The model under review builds one solid part; all positions refer to its coordinate system, in mm. Face numbers are marked on the shaded views. A direction names the side the tool comes from. Coordinates: 2 decimals unless noted, no trailing zeros. Loops run counter-clockwise (first coordinate to the right, second up) from the corner with the lowest first, then second, coordinate; pieces in that order, holes last. Notation, with made-up numbers: (-11.5, 74) - (2.5, 74) arc R19 ccw to (2.5, 107) - close; hole circle Ø3 at (26, 40). An arc over 180 degrees is marked (long way). Use a Markdown table: item, result. Add a question column.
1) Clearance check with flat-ended pins moving along their axes: pin 1 (3 mm diameter, centred on x = -34, z = -34, fed in from +Y); pin 2 (1 mm diameter, centred on y = 7.5, z = 30, fed in from -X). State where each tip first meets the part, or that it passes through.
2) For the marked faces 1 and 2, list the 3-axis set-ups (+Z, -Z, +X, -X, +Y, -Y) from which the entire face can be reached by the end or side of a thin tool; tool diameter is ignored.
3) Add section A-A, the plane z = 34. Give the boundary of the cut face in (x, y), and give its area (3 significant figures).
4) Add section B-B, the plane x = 34. Give the boundary of the cut face in (y, z).
5) To check wall thickness, follow L1, parallel to X at y = 0.4, z = 34; L2, parallel to Z at x = 35, y = 6.75; L3, parallel to Y at x = 31.5, z = -31.5. State the ranges of each line that lie inside material, in increasing order. Write a range as [from, to].
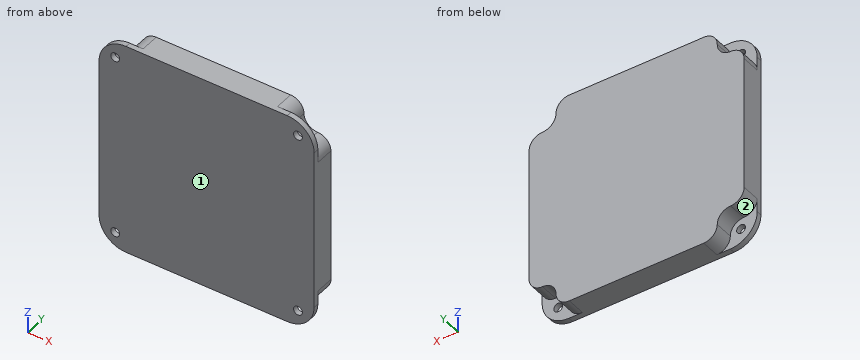
```python
from build123d import *

# Parameters (mm, degrees)
SKETCH_1_R      = 1.65
EXTRUDE_1_DEPTH = 2
EXTRUDE_2_DEPTH = 7
FILLET_1_R      = 5


with BuildPart() as part:
    # 草图1 → 凸台-拉伸1 (new body)
    with BuildSketch(Plane(origin=(0, 0, 0), x_dir=(1, 0, 0), z_dir=(0, 1, 0))):
        with BuildLine():
            Line((-30, -40), (30, -40))
            ThreePointArc((30, -40), (37.071067812, -37.071067812), (40, -30))
            Line((40, -30), (40, 30))
            ThreePointArc((40, 30), (37.071067812, 37.071067812), (30, 40))
            Line((30, 40), (-30, 40))
            ThreePointArc((-30, 40), (-37.071067812, 37.071067812), (-40, 30))
            Line((-40, 30), (-40, -30))
            ThreePointArc((-40, -30), (-37.071067812, -37.071067812), (-30, -40))
        make_face()
        with Locations(Location((-34, 34, 0), (0, 0, 270))):
            Circle(SKETCH_1_R, mode=Mode.SUBTRACT)
        with Locations(Location((-34, -34, 0), (0, 0, 90))):
            Circle(SKETCH_1_R, mode=Mode.SUBTRACT)
        with Locations(Location((34, 34, 0), (0, 0, 90))):
            Circle(SKETCH_1_R, mode=Mode.SUBTRACT)
        with Locations(Location((34, -34, 0), (0, 0, 270))):
            Circle(SKETCH_1_R, mode=Mode.SUBTRACT)
    extrude(amount=EXTRUDE_1_DEPTH)

    # 草图2 → 凸台-拉伸2 (add)
    with BuildSketch(Plane(origin=(0, 2, 0), x_dir=(1, 0, 0), z_dir=(0, 1, 0))):
        Polygon((-30, 40), (-30, 30), (-40, 30), (-40, -30), (-30, -30), (-30, -40), (30, -40), (30, -30), (40, -30), (40, 30), (30, 30), (30, 40), align=None)
    extrude(amount=EXTRUDE_2_DEPTH)

    # 圆角1
    fillet_1_edges = [part.edges().sort_by_distance(p)[0] for p in [
        (-40, 5.5, -30),
        (-30, 5.5, -30),
        (-30, 5.5, -40),
        (30, 5.5, -40),
        (30, 5.5, -30),
        (40, 5.5, -30),
        (40, 5.5, 30),
        (30, 5.5, 30),
        (30, 5.5, 40),
        (-40, 5.5, 30),
        (-30, 5.5, 30),
        (-30, 5.5, 40),
    ]]
    fillet(fillet_1_edges, radius=FILLET_1_R - 0.0001)  # a hair under: the kernel refuses the full size


solid = part.part
```
From the geometry:
| question | item | result |
|---|---|---|
| 1 | pin 1 | passes through |
| 1 | pin 2 | stops at x = -37.18 |
| 2 | face 1 | +Z, -Z, +X, -X, -Y |
| 2 | face 2 | -Z, -X, +Y |
| 3 | outline | (-39.17, 0) - (-35.65, 0) - (-35.65, 2) - (-39.17, 2) - close; (-32.35, 0) - (32.35, 0) - (32.35, 2) - (30.1, 2) - (30.1, 9) - (-30.1, 9) - (-30.1, 2) - (-32.35, 2) - close; (35.65, 0) - (39.17, 0) - (39.17, 2) - (35.65, 2) - close |
| 3 | area | 565 mm^2 |
| 4 | outline | (0, -39.17) - (2, -39.17) - (2, -35.65) - (0, -35.65) - close; (0, -32.35) - (2, -32.35) - (2, -30.1) - (9, -30.1) - (9, 30.1) - (2, 30.1) - (2, 32.35) - (0, 32.35) - close; (0, 35.65) - (2, 35.65) - (2, 39.17) - (0, 39.17) - close |
| 5 | L1 | x = [-39.17, -35.65], [-32.35, 32.35], [35.65, 39.17] |
| 5 | L2 | z = [-30, 30] |
| 5 | L3 | y = [0, 2] |
